Read the model definition and answer for the solid it produces. Units are mm, in the model's axes. Round coordinates to 2 decimals unless told otherwise and drop trailing zeros. Order: outer loops, then holes, each group sorted by start corner. A loop starts at its lowest first (then second) coordinate and runs counter-clockwise, first axis right, second up. Notation, with made-up numbers: M 58,29.25 L 102,29.25 A28 ccw 102,47.25 Z; hole C 10.5,-17 d7. An arc over 180 degrees is marked long. Use one line per item in the form item = value. Start each with the question number.
from build123d import *

# Parameters (mm, degrees)
F3_W     = 33.02
F3_H     = 33.02
F4_DEPTH = 25.4
F5_T     = -0.5


with BuildPart() as f1:
    # F0 (on Front) → F1 (revolve)
    with BuildSketch(Plane.XZ):
        with BuildLine():
            Line((0, 38.1), (0, -38.1))
            ThreePointArc((0, -38.1), (38.1, 0), (0, 38.1))
        make_face()
    revolve(axis=Axis((0, 0, 0), (0, 0, -1)))

    # F3 (on offset) → F4 (cut)
    with BuildSketch(Plane.XY.offset(35.56)):
        Rectangle(F3_W, F3_H)
    extrude(amount=F4_DEPTH, mode=Mode.SUBTRACT)

    # F5
    f5_openings = [f1.faces().sort_by_distance(p)[0] for p in [
        (0, 0, 35.56),
    ]]
    offset(amount=F5_T, openings=f5_openings)


solid = f1.part
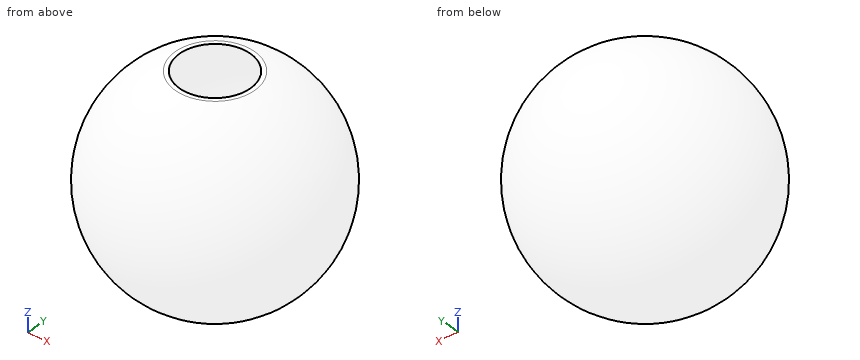
Item 1: Section A-A (x = -25) is taken. Write down the section's boundary in (y, z), and give its area (3 significant figures).
Item 2: Section B-B (x = 3) is taken. Write down the section's boundary in (y, z), and give its area (3 significant figures).
Item 3: Given P1, Ø4, axis at x = -18.5, z = -23, coming from the -Y side; P2, Ø2, axis at x = 19, z = 17, coming from the +Y side; P3, Ø1.5, axis at y = -8, z = -4, coming from the -X side, each flat-ended and moving along its own axis, determine where each tip first touches the part or whether it passes through.
Item 4: Section D-D (x = -7) is taken. Write down the section's boundary in (y, z), and give its area (3 significant figures).
Item 5: Find the intervals of material crossed by L1, parallel to Y at x = 26, z = 6; L2, parallel to Y at x = 8.5, z = 17; L3, parallel to Z at x = 27.5, y = 8, in increasing order. Write a range as [from, to].
The answers:
q1.outline = C 0,0 d57.5; hole C 0,0 d56.17
q1.area = 119 mm²
q2.outline = M -13.35,35.56 A37.98 ccw long 13.35,35.56 L 11.84,35.56 A37.48 cw long -11.84,35.56 Z
q2.area = 106 mm²
q3.P1 = -26.35
q3.P2 = 29.18
q3.P3 = -37.21
q4.outline = M -11.75,35.56 A37.45 ccw long 11.75,35.56 L 10.01,35.56 A36.94 cw long -10.01,35.56 Z
q4.area = 108 mm²
q5.L1 = [-27.2, -26.49], [26.49, 27.2]
q5.L2 = [-33.02, -32.44], [32.44, 33.02]
q5.L3 = [-25.13, -24.36], [24.36, 25.13]
